Design review of the part built by this model. Coordinates are the model's own, in mm. A direction names the side the tool comes from. Round coordinates to 2 decimals unless told otherwise and drop trailing zeros. Write each loop counter-clockwise with the first axis right and the second up, starting at its lowest first coordinate (ties: lowest second). Pieces come first, ordered by that corner, then holes. Notation, with made-up numbers: (-29, 30) - (-25, 30) arc R12 cw to (-25, 34) - close; hole circle Ø3 at (-9, 7). An arc over 180 degrees is marked (long way). Use one line per item in the form item = value.
```python
from build123d import *

# Parameters (mm, degrees)
F0_W     = 535
F0_H     = 330
F0_W_2   = 520
F0_H_2   = 313
F1_DEPTH = 8.5
F2_DEPTH = 27
F2_TAPER = 5
F3_W     = 244
F3_H     = 133
F4_DEPTH = 48.5
F5_R     = 5
F6_R     = 10
F7_SIZE  = 3


with BuildPart() as f1:
    # F0 (on Top) → F1 (new body)
    with BuildSketch(Plane.XY):
        Rectangle(F0_W, F0_H)
        Rectangle(F0_W_2, F0_H_2, mode=Mode.SUBTRACT)
        Rectangle(F0_W_2, F0_H_2)
    extrude(amount=F1_DEPTH)

    # F0 (on Top) → F2 (join)
    with BuildSketch(Plane.XY):
        Rectangle(F0_W_2, F0_H_2)
    extrude(amount=-F2_DEPTH, taper=F2_TAPER)

    # F3 (on face) → F4 (join)
    with BuildSketch(Plane(origin=(0, 0, -27), x_dir=(1, 0, 0), z_dir=(0, 0, -1))):
        with Locations((0, -80.3621939152)):
            Rectangle(F3_W, F3_H)
    extrude(amount=F4_DEPTH)

    # F5
    f5_edges = [f1.edges().sort_by_distance(p)[0] for p in [
        (267.5, 165, 4.25),
        (-267.5, 165, 4.25),
        (-267.5, -165, 4.25),
        (267.5, -165, 4.25),
    ]]
    fillet(f5_edges, radius=F5_R)

    # F6
    f6_edges = [f1.edges().sort_by_distance(p)[0] for p in [
        (258.818903, -155.318903, -13.5),
        (258.818903, 155.318903, -13.5),
        (-258.818903, 155.318903, -13.5),
        (-258.818903, -155.318903, -13.5),
    ]]
    fillet(f6_edges, radius=F6_R)

    # F7
    f7_edges = [f1.edges().sort_by_distance(p)[0] for p in [
        (0, -165, 8.5),
    ]]
    chamfer(f7_edges, length=F7_SIZE)


solid = f1.part
```
Q1. Machinability: for faces 1 (the flat face through (-122, 81, -51)), 2 (the flat face through (-2, 79, -75.5)), which of the approach directions +Z, -Z, +X, -X, +Y, -Y give a long, thin tool a straight path to every point of the face, cutting with its end or side? Answer none if there is none.
Calculated:
face_1 = -Z, -X, +Y, -Y
face_2 = -Z, +X, -X, +Y, -Y
Q2. We need section A-A on z = -63. Write out the cut boundary in (x, y).
Calculated:
outline = (-122, 13.86) - (122, 13.86) - (122, 146.86) - (-122, 146.86) - close
Q3. For P1, Ø24, axis at y = 87, z = -57.5, coming from the +X side; P2, Ø6, axis at x = -190.5, z = -14.5, coming from the +Y side; P3, Ø1, axis at x = -23, z = -37, coming from the +Y side, all flat-tipped, find the tip position at first contact; note any pin that passes through.
Calculated:
P1 = 122
P2 = 155.49
P3 = 146.86
Q4. Draft analysis for pull direction Y (two halves, no side actions). For faces 3 (the flat face through (-2, 13.862, -51)), 4 (the flat face through (-2, 146.862, -51)), 5 (the flat face through (122, 81, -51)), state which applies: released by +Y, released by -Y, zero draft, split by the parting line, or undercut.
Calculated:
face_3 = released by -Y
face_4 = released by +Y
face_5 = zero draft
Q5. To check wall thickness, follow line 1 along X through (y, z) = (120, -53); line 2 along Z through (x, y) = (-235, -59.5); line 3 along Y through (x, z) = (-23, -62.5). State the ranges of each line that lie inside material, in increasing order. Write a range as from..to.
Calculated:
line_1 = -122..122
line_2 = -27..8.5
line_3 = 13.86..146.86
